```python
from build123d import *

# Parameters (mm, degrees)
EXTRUDE_THIN2_DEPTH                                 = 31.75
CBORE_FOR_00_BINDING_HEAD_MACHINE_SCREW_D           = 6.35
CBORE_FOR_00_BINDING_HEAD_MACHINE_SCREW_CBORE_D     = 19.05
CBORE_FOR_00_BINDING_HEAD_MACHINE_SCREW_CBORE_DEPTH = 3.81
SKETCH14_R                                          = 5.08
CUT_EXTRUDE1_DEPTH                                  = 91.918163752
LPATTERN1_COUNT                                     = 2
LPATTERN1_PITCH                                     = 38.1
LPATTERN1_COUNT_DIR2                                = 2
LPATTERN1_PITCH_DIR2                                = 114.3
FILLET1_R                                           = 2.54


with BuildPart() as part:
    # Sketch3 → Extrude-Thin2 (new, symmetric)
    with BuildSketch(Plane.XY):
        Polygon((-76.2, 38.1), (-38.1, 38.1), (-38.1, 76.2), (38.1, 76.2), (38.1, 38.1), (76.2, 38.1), (76.2, 31.75), (31.75, 31.75), (31.75, 69.85), (-31.75, 69.85), (-31.75, 31.75), (-76.2, 31.75), align=None)
    extrude(amount=EXTRUDE_THIN2_DEPTH, both=True)

    # CBORE for #00 Binding Head Machine Screw1 (through all)
    with Locations(Plane(origin=(0, 76.2, 0), x_dir=(1, 0, 0), z_dir=(0, 1, 0))):
        with Locations((0, 0)):
            CounterBoreHole(CBORE_FOR_00_BINDING_HEAD_MACHINE_SCREW_D / 2, CBORE_FOR_00_BINDING_HEAD_MACHINE_SCREW_CBORE_D / 2, CBORE_FOR_00_BINDING_HEAD_MACHINE_SCREW_CBORE_DEPTH)

    # Sketch14 → Cut-Extrude1 (cut, through all)
    with BuildSketch(Plane(origin=(0, 38.1, 0), x_dir=(1, 0, 0), z_dir=(0, 1, 0))):
        with Locations(Location((-57.15, -19.05, 0), (0, 0, 270))):
            Circle(SKETCH14_R)
    cut_extrude1 = extrude(amount=-CUT_EXTRUDE1_DEPTH, mode=Mode.SUBTRACT)

    # LPattern1: Cut-Extrude1 2 × 2
    with Locations(*[(j * LPATTERN1_PITCH_DIR2, 0, -i * LPATTERN1_PITCH) for i in range(LPATTERN1_COUNT) for j in range(LPATTERN1_COUNT_DIR2) if (i, j) != (0, 0)]):
        add(cut_extrude1, mode=Mode.SUBTRACT)

    # Fillet1
    fillet1_edges = [part.edges().sort_by_distance(p)[0] for p in [
        (-57.15, 38.1, -31.75),
        (-38.1, 57.15, -31.75),
        (0, 76.2, -31.75),
        (57.15, 38.1, 31.75),
        (38.1, 57.15, -31.75),
        (57.15, 38.1, -31.75),
        (38.1, 57.15, 31.75),
        (-76.2, 38.1, 0),
        (-38.1, 76.2, 0),
        (38.1, 76.2, 0),
        (76.2, 38.1, 0),
        (0, 76.2, 31.75),
        (-38.1, 57.15, 31.75),
        (-57.15, 38.1, 31.75),
        (-76.2, 34.925, 31.75),
    ]]
    fillet(fillet1_edges, radius=FILLET1_R)


solid = part.part
```
CAD build for the part. Positions are in the model's coordinates, mm. A direction names the side the tool comes from. Round coordinates to 2 decimals unless told otherwise and drop trailing zeros. Loops run counter-clockwise (first coordinate to the right, second up) from the corner with the lowest first, then second, coordinate; pieces in that order, holes last. Notation, with made-up numbers: M 73,-10.75 L 102,-10.75 A25 ccw 102,20.25 Z; hole C 19.5,-24.5 d11. An arc over 180 degrees is marked long. Return JSON: item names as keys, results as strings. Group by question number.
(1) Mould opens along Z. For faces 1 (the flat face through (-56, 38.1, 0)), 2 (the flat face through (13, 70, 31.75)), 3 (the cylindrical face through (-61.66, 34.97, -16.71)) say: +Z half, -Z half, draft (parallel to the pull), parting line (faces both ways), or undercut.
(2) Saw through at D-D, the plane z = 26. List the corners of the cut face in (x, y).
(3) Saw through at A-A, the plane y = 43.5. List the corners of the cut face in (x, z), and give its area (3 significant figures).
(4) Wall check: probe 1 along Z at (x, y) = (-57, 33); probe 2 along X at (y, z) = (45.5, -18); probe 3 along Z at (x, y) = (0, 71.05) (3 decimals). Give the ranges that are in metal, low to high. Write a range as [from, to].
(5) Saw through at C-C, the plane x = -57.15. List the corners of the cut face in (y, z), and give its area (3 significant figures).
(6) Drop flat-ended pins along their axis: P1, Ø19, axis at x = 5.5, z = 7.5, coming from the -Y side; P2, Ø11.5, axis at y = 45.5, z = 9.5, coming from the -X side; P3, Ø10, axis at x = 45.5, z = -17, coming from the +Y side. Give the stop position or say it passes through.
(7) Saw through at B-B, the plane z = -19.05. List the corners of the cut face in (x, y), and give its area (3 significant figures).
(8) Tool access for faces 4 (the flat face through (76.2, 34, 0)), 5 (the flat face through (-7, 69.85, 0)), 6 (the cylindrical face through (58.676, 34.969, -14.205)), 7 (the flat face through (4, 72.39, 0)), 8 (the flat face through (38.1, 56, 0)): list every direction of +Z, -Z, +X, -X, +Y, -Y with a clear straight run to the whole face (end or side of a thin tool).
Answer list:
{
 "1": {"face 1": "draft", "face 2": "+Z half", "face 3": "undercut"},
 "2": {"outline": "M -76.2,31.75 L -31.75,31.75 L -31.75,69.85 L 31.75,69.85 L 31.75,31.75 L 76.2,31.75 L 76.2,35.56 A2.54 ccw 73.66,38.1 L 38.1,38.1 L 38.1,73.66 A2.54 ccw 35.56,76.2 L -35.56,76.2 A2.54 ccw -38.1,73.66 L -38.1,38.1 L -73.66,38.1 A2.54 ccw -76.2,35.56 Z"},
 "3": {"outline": "M -38.1,-29.21 A2.54 ccw -35.56,-31.75 L -31.75,-31.75 L -31.75,31.75 L -35.56,31.75 A2.54 ccw -38.1,29.21 Z; M 31.75,-31.75 L 35.56,-31.75 A2.54 ccw 38.1,-29.21 L 38.1,29.21 A2.54 ccw 35.56,31.75 L 31.75,31.75 Z", "area": "801 mm2"},
 "4": {"probe 1": "[-31.75, -24.13], [-13.97, 13.97], [24.13, 31.75]", "probe 2": "[-38.1, -31.75], [31.75, 38.1]", "probe 3": "[-31.75, -3.175], [3.175, 31.75]"},
 "5": {"outline": "M 31.75,-31.75 L 35.56,-31.75 A2.54 ccw 38.1,-29.21 L 38.1,-24.13 L 31.75,-24.13 Z; M 31.75,-13.97 L 38.1,-13.97 L 38.1,13.97 L 31.75,13.97 Z; M 31.75,24.13 L 38.1,24.13 L 38.1,29.21 A2.54 ccw 35.56,31.75 L 31.75,31.75 Z", "area": "271 mm2"},
 "6": {"P1": "y = 69.85", "P2": "x = -38.1", "P3": "y = 38.1"},
 "7": {"outline": "M -76.2,31.75 L -62.23,31.75 L -62.23,38.1 L -73.66,38.1 A2.54 ccw -76.2,35.56 Z; M -52.07,31.75 L -31.75,31.75 L -31.75,69.85 L 31.75,69.85 L 31.75,31.75 L 52.07,31.75 L 52.07,38.1 L 38.1,38.1 L 38.1,73.66 A2.54 ccw 35.56,76.2 L -35.56,76.2 A2.54 ccw -38.1,73.66 L -38.1,38.1 L -52.07,38.1 Z; M 62.23,31.75 L 76.2,31.75 L 76.2,35.56 A2.54 ccw 73.66,38.1 L 62.23,38.1 Z", "area": "1,320 mm2"},
 "8": {"face 4": "+Z, -Z, +X, +Y, -Y", "face 5": "+Z, -Z, -Y", "face 6": "+Y, -Y", "face 7": "+Y", "face 8": "+Z, -Z, +X, +Y"}
}
